Geometry: final body of the model. Coordinates: model frame, mm. Face numbers are marked on the shaded views. A direction names the side the tool comes from. Coordinates: 2 decimals unless noted, no trailing zeros. Write each loop counter-clockwise with the first axis right and the second up, starting at its lowest first coordinate (ties: lowest second). Pieces come first, ordered by that corner, then holes. Notation, with made-up numbers: M 23,-17 L 63,-17 A32 ccw 63,11 Z; hole C 36,88 d11. An arc over 180 degrees is marked long. Write item = value, one per line. Start each with the question number.
Item 1: Ray query, L1, parallel to Y at x = 0.75, z = 128.25; L2, parallel to X at y = 47, z = 150. Return the intervals inside material, ascending. Write a range as [from, to].
Item 2: Section B-B on z = 22.5. Output: boundary loops of the cut face in (x, y).
Item 3: First-contact query: pin 1 Ø14.5 at (x, z) = (28.5, 79.5) entering from +Y; pin 2 Ø8 at (x, y) = (8, 37) entering from -Z; pin 3 Ø24 at (y, z) = (26.5, 46) entering from +X. Flat tips, straight axial feed; report the tip coordinate or a pass-through.
Item 4: Section A-A on y = 19.25. Output: boundary loops of the cut face in (x, z), plus the area to 3 significant figures.
Item 5: Reachability of the marked faces 1 and 2 from +Z, -Z, +X, -X, +Y, -Y: full face, straight path, thin tool, end or side. Return the list, or none.
Item 6: Section C-C on x = 21. Output: boundary loops of the cut face in (y, z).
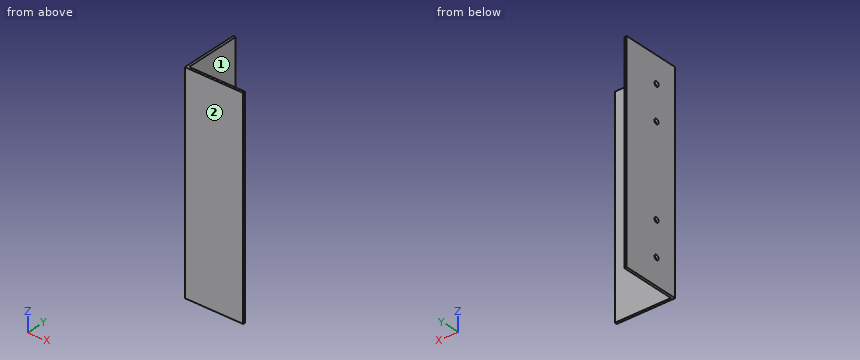
from build123d import *

# Parameters (mm, degrees)
BOSS_EXTRUDE1_DEPTH = 180
SKETCH2_R           = 2.1
CUT_EXTRUDE1_DEPTH  = 5


with BuildPart() as part:
    # Sketch1 → Boss-Extrude1 (new body)
    with BuildSketch(Plane.XY):
        Polygon((0, 0), (50, 0), (50, 2), (2, 2), (2, 50), (0, 50), align=None)
    extrude(amount=BOSS_EXTRUDE1_DEPTH)

    # Sketch2 → Cut-Extrude1 (cut, symmetric)
    with BuildSketch(Plane(origin=(0, 0, 0), x_dir=(0, 0, -1), z_dir=(1, 0, 0))):
        with Locations((-22.5, 19.25)):
            Circle(SKETCH2_R)
        with Locations((-51.75, 19.25)):
            Circle(SKETCH2_R)
        with Locations((-128.25, 19.25)):
            Circle(SKETCH2_R)
        with Locations((-157.5, 19.25)):
            Circle(SKETCH2_R)
    extrude(amount=CUT_EXTRUDE1_DEPTH, both=True, mode=Mode.SUBTRACT)


solid = part.part
Responses:
q1.L1 = [0, 17.15], [21.35, 50]
q1.L2 = [0, 2]
q2.outline = M 0,0 L 50,0 L 50,2 L 2,2 L 2,17.15 L 0,17.15 Z; M 0,21.35 L 2,21.35 L 2,50 L 0,50 Z
q3.pin_1 = 2
q3.pin_2 = through
q3.pin_3 = 2
q4.outline = M 0,0 L 2,0 L 2,20.4 L 0,20.4 Z; M 0,24.6 L 2,24.6 L 2,49.65 L 0,49.65 Z; M 0,53.85 L 2,53.85 L 2,126.15 L 0,126.15 Z; M 0,130.35 L 2,130.35 L 2,155.4 L 0,155.4 Z; M 0,159.6 L 2,159.6 L 2,180 L 0,180 Z
q4.area = 326 mm²
q5.face_1 = +Z, -Z, +X, +Y
q5.face_2 = +Z, -Z, +X, -X, -Y
q6.outline = M 0,0 L 2,0 L 2,180 L 0,180 Z
